from build123d import *

# Parameters (mm, degrees)
SKETCH1_W           = 3.45
SKETCH1_H           = 1.1
BOSS_EXTRUDE3_DEPTH = 0.7
SKETCH1_3_W         = 3.45
SKETCH1_3_H         = 1.1
CUT_EXTRUDE1_DEPTH  = 0.35
SKETCH2_W           = 3.95
SKETCH2_H           = 0.9
BOSS_EXTRUDE4_DEPTH = 0.35
BOSS_EXTRUDE5_DEPTH = 0.35
BOSS_EXTRUDE6_DEPTH = 3.25
FILLET1_R           = 0.5
FILLET2_R           = 0.45
FILLET3_R           = 0.25


with BuildPart() as part:
    # Sketch1 → Boss-Extrude3 (new body)
    with BuildSketch(Plane.XY):
        with Locations((4.075, 0)):
            Rectangle(SKETCH1_W, SKETCH1_H)
        with Locations((-4.075, 0)):
            Rectangle(SKETCH1_W, SKETCH1_H)
        Polygon((-2.35, 0.55), (-5.8, 0.55), (-5.8, 2.415), (5.8, 2.415), (5.8, 0.55), (2.35, 0.55), (2.35, -0.55), (5.8, -0.55), (5.8, -2.415), (-5.8, -2.415), (-5.8, -0.55), (-2.35, -0.55), align=None)
    extrude(amount=BOSS_EXTRUDE3_DEPTH)

    # Sketch1<3> → Cut-Extrude1 (cut)
    with BuildSketch(Plane.XY):
        with Locations((4.075, 0)):
            Rectangle(SKETCH1_3_W, SKETCH1_3_H)
        with Locations((-4.075, 0)):
            Rectangle(SKETCH1_3_W, SKETCH1_3_H)
    extrude(amount=CUT_EXTRUDE1_DEPTH, mode=Mode.SUBTRACT)

    # Sketch2 → Boss-Extrude4 (add)
    with BuildSketch(Plane.XY):
        with Locations((4.425, 0)):
            Rectangle(SKETCH2_W, SKETCH2_H)
        with Locations((-4.425, 0)):
            Rectangle(SKETCH2_W, SKETCH2_H)
    extrude(amount=BOSS_EXTRUDE4_DEPTH)

    # Sketch3 → Boss-Extrude5 (add)
    with BuildSketch(Plane.XY.offset(0.7)):
        with BuildLine():
            Line((-3.2, 2.35), (3.2, 2.35))
            ThreePointArc((3.2, 2.35), (5.55, 0), (3.2, -2.35))
            Line((3.2, -2.35), (-3.2, -2.35))
            ThreePointArc((-3.2, -2.35), (-5.55, 0), (-3.2, 2.35))
        make_face()
    extrude(amount=BOSS_EXTRUDE5_DEPTH)

    # Sketch4 → Boss-Extrude6 (add)
    with BuildSketch(Plane.XY.offset(1.05)):
        with BuildLine():
            Line((-3.2, 1.9), (3.2, 1.9))
            ThreePointArc((3.2, 1.9), (5.1, 0), (3.2, -1.9))
            Line((3.2, -1.9), (-3.2, -1.9))
            ThreePointArc((-3.2, -1.9), (-5.1, 0), (-3.2, 1.9))
        make_face()
    extrude(amount=BOSS_EXTRUDE6_DEPTH)

    # Fillet1
    fillet1_edges = [part.edges().sort_by_distance(p)[0] for p in [
        (0, 1.9, 4.3),
        (-5.1, 0, 4.3),
        (0, -1.9, 4.3),
        (5.1, 0, 4.3),
    ]]
    fillet(fillet1_edges, radius=FILLET1_R)

    # Fillet2
    fillet2_edges = [part.edges().sort_by_distance(p)[0] for p in [
        (-5.1, 0, 1.05),
        (0, -1.9, 1.05),
        (5.1, 0, 1.05),
        (0, 1.9, 1.05),
    ]]
    fillet(fillet2_edges, radius=FILLET2_R - 0.0001)  # a hair under: the kernel refuses the full size

    # Fillet3
    fillet3_edges = [part.edges().sort_by_distance(p)[0] for p in [
        (-5.8, 2.415, 0.35),
        (5.8, 2.415, 0.35),
        (5.8, -2.415, 0.35),
        (-5.8, -2.415, 0.35),
    ]]
    fillet(fillet3_edges, radius=FILLET3_R)


solid = part.part
Build history of the part. All positions in model axes, mm. A direction names the side the tool comes from. Give positions to 0.01 mm unless a question says otherwise; leave off trailing zeros. Write each loop counter-clockwise with the first axis right and the second up, starting at its lowest first coordinate (ties: lowest second). Pieces come first, ordered by that corner, then holes. Notation, with made-up numbers: (80.25, -25.75) - (131.25, -25.75) arc R16 cw to (131.25, -13.75) - close; hole circle Ø6 at (33.25, -27.75). An arc over 180 degrees is marked (long way). Use one line per item in the form item = value. Start each with the question number.
1. Band-saw the part on B-B on z = 0.5. Write the cut outline in (x, y) (3 decimals), plus the area to 3 significant figures.
2. 3-axis set-ups, long thin cutter, end or side, ignore diameter. For faces 1 (the face through (5.55, 0.05, 0.87)), 2 (the face through (-5.1, 0, 2.6)), 3 (the face through (0, -1.9, 3)): which of +Z, -Z, +X, -X, +Y, -Y reach the whole face in a straight line?
3. Drop flat-ended pins along their axis: pin 1 Ø1.2 at (x, z) = (-0.5, 2.5) entering from +Y; pin 2 Ø1.2 at (x, z) = (-1, 2) entering from -Y; pin 3 Ø1 at (y, z) = (1, 0.5) entering from -X. Give the stop position or say it passes through.
4. Probe line 1 (Y direction, x = 1, z = 1.9); line 2 (X direction, y = 0, z = 3.15); line 3 (X direction, y = -0.4, z = 0.5). List the from-to ranges inside material, lowest first. Write a range as [from, to].
5. Band-saw the part on D-D on z = 2.6. Write the cut outline in (x, y), plus the area to 3 significant figures.
Conclusion:
q1.outline = (-5.8, -2.165) arc R0.25 ccw to (-5.55, -2.415) - (5.55, -2.415) arc R0.25 ccw to (5.8, -2.165) - (5.8, 2.165) arc R0.25 ccw to (5.55, 2.415) - (-5.55, 2.415) arc R0.25 ccw to (-5.8, 2.165) - close
q1.area = 56.0 mm²
q2.face_1 = +Z, +X
q2.face_2 = +Z, -X
q2.face_3 = +Z, +X, -X, -Y
q3.pin_1 = 1.9
q3.pin_2 = -1.91
q3.pin_3 = -5.8
q4.line_1 = [-1.9, 1.9]
q4.line_2 = [-5.1, 5.1]
q4.line_3 = [-5.8, 5.8]
q5.outline = (-3.2, -1.9) - (3.2, -1.9) arc R1.9 ccw to (3.2, 1.9) - (-3.2, 1.9) arc R1.9 ccw to start
q5.area = 35.7 mm²
